Autodesk Inventor part; units mm, degrees
ref_plane "YZ Plane" through (0, 0, 0) normal (1, 0, 0) x (0, 1, 0)
ref_plane "XZ Plane" through (0, 0, 0) normal (0, 1, 0) x (-1, 0, 0)
ref_plane "XY Plane" through (0, 0, 0) normal (0, 0, 1) x (1, 0, 0)
sketch "Esboço1" plane through (0, 0, 0) normal (1, 0, 0) x (0, 1, 0)
  line L0 (0, 0) -> (6, 0)
  line L1 (6, 0) -> (6, -6)
  line L2 (6, -6) -> (0, -6)
  line L3 (0, -6) -> (0, 0)
  dimension "d0" = 6
  dimension "d1" = 6
extrude "Extrusão1" add sketch "Esboço1" along normal blind 6
sketch "Esboço2" plane through (0, 0, -6) normal (0, -1, 0) x (1, 0, 0)
  line L0 (0, 6) -> (6, 6)
  line L1 (0, 0) -> (6, 0)
  point P0 (3, 3)
hole "Furo1" at (3, 0, -3) direction (0, 1, 0) diameter 3.242 depth 4
sketch "Esboço3" plane through (0, 0, -6) normal (0, 0, -1) x (-1, 0, 0)
  line L0 (0, 0) -> (-6, 0)
  line L1 (0, 6) -> (-6, 6)
  circle A0 centre (-3, 3) radius 2
  dimension "d11" = 4
extrude "Extrusão2" add sketch "Esboço3" along normal blind 2.5
sketch "Esboço4" plane through (3, 3, -8.5) normal (0, 0, -1) x (-1, 0, 0)
  point P0 (3, -3)
  point P1 (0, 0)
sketch "Esboço7" plane through (3, 3, -8.5) normal (0, 0, -1) x (-1, 0, 0)
  circle A0 centre (0, 0) radius 1.5
  point P0 (3, -3)
  dimension "d20" = 3
extrude "Extrusão4" add sketch "Esboço7" along normal blind 2
thread "Rosca2"
fillet "Arredondamento1" radius 1 1 edges at (6, 0, -3)
fillet "Arredondamento2" radius 1 3 edges at (6, 3.5, 0) (5.7071, 0.2929, 0) (2.5, 0, 0)
fillet "Arredondamento3" radius 1 3 edges at (0, 3.5, 0) (0, 0.2929, -0.2929) (0, 0, -3.5)
fillet "Arredondamento4" radius 1 5 edges at (3, 6, 0) (5.7071, 6, -0.2929) (6, 6, -3.5) (0.2929, 6, -0.2929) (0, 6, -3.5)
properties part number "CONECTOR L-F"
Input: part model. Units: mm. Frame: model coordinates. A direction names the side the tool comes from. Coordinates: 2 decimals unless noted, no trailing zeros. Order: outer loops, then holes, each group sorted by start corner. A loop starts at its lowest first (then second) coordinate and runs counter-clockwise, first axis right, second up. Notation, with made-up numbers: M 11.5,-0.5 L 44.5,-0.5 A37 ccw 44.5,37.5 Z; hole C -37.5,71.5 d3. An arc over 180 degrees is marked long. Write item = value, one per line. Start each with the question number.
(1) Section B-B on x = 3. Output: boundary loops of the cut face in (y, z).
(2) First-contact query: P1, Ø1.9, axis at x = 3, z = -3, coming from the -Y side. Flat tip, straight axial feed; report the tip coordinate or a pass-through.
(3) Pull-direction query (X, two-part tool) for faces 1 (the cylindrical face through (2.194, 1.735, -9.486)), 2 (the flat face through (3, 4, -3)), 3 (the flat face through (3, 6, -3)); classes: released by +X, released by -X, zero draft, split by the parting line, or undercut.
(4) Section A-A on y = 3. Output: boundary loops of the cut face in (x, z), and give its area (3 significant figures).
(5) Section D-D on y = 5.4. Output: boundary loops of the cut face in (x, z), and give its area (3 significant figures).
(6) Reachability of faces 4 (the cylindrical face through (5.699, 0.285, -3.465)), 5 (the cylindrical face through (3.986, 2.028, -1.714)), 6 (the cylindrical face through (3, 5, -7)) from +Z, -Z, +X, -X, +Y, -Y: full face, straight path, thin tool, end or side. Return the list, or none.
(7) Section C-C on z = -3. Output: boundary loops of the cut face in (x, y).
(8) Line query: line 1 along X through (y, z) = (3.25, -3); line 2 along Z through (x, y) = (3, 2.65); line 3 along Y through (x, z) = (3, -8). Output: solid intervals per line, ascending. Write a range as [from, to].
Result set:
q1.outline = M 0,-6 L 1,-6 L 1,-8.5 L 1.5,-8.5 L 1.5,-10.5 L 4.5,-10.5 L 4.5,-8.5 L 5,-8.5 L 5,-6 L 6,-6 L 6,-1 A1 ccw 5,0 L 1,0 A1 ccw 0,-1 L 0,-1.38 L 4,-1.38 L 4,-4.62 L 0,-4.62 Z
q2.P1 = 4
q3.face_1 = split by the parting line
q3.face_2 = undercut
q3.face_3 = zero draft
q4.outline = M 0,-6 L 1,-6 L 1,-8.5 L 1.5,-8.5 L 1.5,-10.5 L 4.5,-10.5 L 4.5,-8.5 L 5,-8.5 L 5,-6 L 6,-6 L 6,-1 A1 ccw 5,0 L 1,0 A1 ccw 0,-1 Z; hole C 3,-3 d3.24
q4.area = 43.3 mm²
q5.outline = M 0.08,-6 L 5.92,-6 L 5.92,-1 A0.92 ccw 5,-0.08 L 1,-0.08 A0.92 ccw 0.08,-1 Z
q5.area = 34.2 mm²
q6.face_4 = +Z, -Z, +X, -Y
q6.face_5 = -Y
q6.face_6 = -Z
q7.outline = M 0,1 A1 ccw 1,0 L 1.38,0 L 1.38,4 L 4.62,4 L 4.62,0 L 5,0 A1 ccw 6,1 L 6,5 A1 ccw 5,6 L 1,6 A1 ccw 0,5 Z
q8.line_1 = [0, 1.38], [4.62, 6]
q8.line_2 = [-10.5, -4.62], [-1.38, 0]
q8.line_3 = [1, 5]
